Input: part model. Units: mm. Frame: model coordinates. A direction names the side the tool comes from. Round coordinates to 2 decimals unless told otherwise and drop trailing zeros. Write each loop counter-clockwise with the first axis right and the second up, starting at its lowest first coordinate (ties: lowest second). Pieces come first, ordered by that corner, then holes. Notation, with made-up numbers: (31, 72.5) -> (77, 72.5) arc R26 ccw to (77, 108.5) -> close; hole circle Ø4 at (15.25, 32). An arc over 180 degrees is marked (long way). Write item = value, one per line. Start each with the question number.
Autodesk Inventor part; units mm, degrees
ref_plane "YZ Plane" through (0, 0, 0) normal (1, 0, 0) x (0, 1, 0)
ref_plane "XZ Plane" through (0, 0, 0) normal (0, 1, 0) x (-1, 0, 0)
ref_plane "XY Plane" through (0, 0, 0) normal (0, 0, 1) x (1, 0, 0)
sketch "Skizze1" plane through (0, 0, 0) normal (0, 0, 1) x (1, 0, 0)
  circle A0 centre (0, 0) radius 12.5
  dimension "d0" = 25
extrude "Extrusion1" add sketch "Skizze1" along normal blind 4
sketch "Skizze2" plane through (0, 0, 4) normal (0, 0, 1) x (1, 0, 0)
  circle A0 centre (0, 0) radius 12.5
  circle A1 centre (0, 0) radius 5.5
  dimension "d3" = 11
extrude "Extrusion2" add sketch "Skizze2" along normal blind 9 contours A1
sketch "Skizze3" plane through (0, 0, 13) normal (0, 0, 1) x (1, 0, 0)
  circle A0 centre (0, 0) radius 5.5
  circle A1 centre (0, 0) radius 4
  dimension "d6" = 8
extrude "Extrusion3" add sketch "Skizze3" along normal blind 9 contours A1
sketch "Skizze4" plane through (0, 0, 0) normal (0, 0, -1) x (-1, 0, 0)
  circle A0 centre (0, 0) radius 12.5
  line L0 (17.5, 0) -> (-17.5, 0)
  line L1 (0, -17.5) -> (0, 17.5)
  circle A1 centre (0, 0) radius 9
  line L2 (7.7942, -4.5) -> (0, 0)
  line L3 (0, 0) -> (-7.7942, -4.5)
  point P0 (0, 9)
  dimension "d9" = 18
  dimension "d10" = 120
  dimension "d11" = 120
hole "Bohrung1" at (0, 9, 0) at (-7.7942, -4.5, 0) at (7.7942, -4.5, 0) direction (0, 0, 1) diameter 2.459 end through all
chamfer "Fase1" distance 0.5 angle 45 1 edges at (-4, 0, 22)
sketch "Skizze5" plane through (0, 0, 0) normal (1, 0, 0) x (0, 1, 0)
  line L0 (-4, 13) -> (4, 13)
  line L1 (4, 21.5) -> (-4, 21.5)
  line L2 (4, 13) -> (4, 21.5)
  line L3 (0, -4.3) -> (0, 25.8)
  line L4 (4, 20.9) -> (3.8, 20.9)
  line L5 (3.8, 20.9) -> (3.8, 20)
  line L6 (3.8, 20) -> (4, 20)
  line L7 (4, 20) -> (4, 20.9)
  point P0 (0, 0)
  dimension "d31" = 7
  dimension "d32" = 0.9
  dimension "d33" = 7.6
revolve "Umdrehung1" cut sketch "Skizze5" angle 360 about axis through (0, 0, -10) along (0, 0, 1) contours L6 L5 L4 L2
chamfer "Fase3" distance 1 angle 45 1 edges at (-12.5, 0, 4)
properties part number "1_0204_005"
1. Section D-D (y = -4.5). State how many separate pieces and enclosed holes the cut face has, then the cut area to 3 significant figures.
2. Section C-C (z = 16.75). Output: boundary loops of the cut face in (x, y).
3. Line query: line 1 along Y through (x, z) = (0, 1.6); line 2 along X through (y, z) = (-4.5, 1.6); line 3 along Z through (x, y) = (0.5, 7). Output: solid intervals per line, ascending.
4. Section B-B (y = 0). Output: boundary loops of the cut face in (x, z).
5. Pin query (flat end, axial travel): P1, Ø3, axis at x = 7.79, y = -4.5, coming from the +Z side; P2, Ø1, axis at x = -1.5, z = 14.5, coming from the -Y side; P3, Ø3, axis at x = -2.5, z = 11, coming from the +Y side. Return the tip coordinate at first contact, or that it passes through.
6. Mould query, pull axis Y, two halves, no side actions, for faces 1 (the flat face through (0, 0, 0)), 2 (the cylindrical face through (-8.625, -5.406, 2.028)), 3 (the cylindrical face through (0.167, -3.796, 20.444)). Classes: pulls with the +Y half, pulls with the -Y half, needs draft (parallel to the pull), parting line crosses it, or undercut.
7. Section A-A (x = 0). Output: boundary loops of the cut face in (y, z), then the cut area to 3 significant figures.
8. Reachability of faces 4 (the cylindrical face through (6.963, -5.406, 2.028)), 5 (the cylindrical face through (-0.867, 3.905, 16.451)) from +Z, -Z, +X, -X, +Y, -Y: full face, straight path, thin tool, end or side. Return the list, or none.
Check sheet entries:
q1.separate_pieces = 3
q1.enclosed_holes = 0
q1.area = 129 mm2
q2.outline = circle Ø8 at (0, 0)
q3.line_1 = -12.5 to 7.77, 10.23 to 12.5
q3.line_2 = -11.66 to -9.02, -6.56 to 6.56, 9.02 to 11.66
q3.line_3 = 0 to 4
q4.outline = (-12.5, 0) -> (12.5, 0) -> (12.5, 3) -> (11.5, 4) -> (5.5, 4) -> (5.5, 13) -> (4, 13) -> (4, 20) -> (3.8, 20) -> (3.8, 20.9) -> (4, 20.9) -> (4, 21.5) -> (3.5, 22) -> (-3.5, 22) -> (-4, 21.5) -> (-4, 20.9) -> (-3.8, 20.9) -> (-3.8, 20) -> (-4, 20) -> (-4, 13) -> (-5.5, 13) -> (-5.5, 4) -> (-11.5, 4) -> (-12.5, 3) -> close
q5.P1 = 4
q5.P2 = -3.87
q5.P3 = 5.41
q6.face_1 = needs draft
q6.face_2 = undercut
q6.face_3 = parting line crosses it
q7.outline = (-12.5, 0) -> (7.77, 0) -> (7.77, 4) -> (5.5, 4) -> (5.5, 13) -> (4, 13) -> (4, 20) -> (3.8, 20) -> (3.8, 20.9) -> (4, 20.9) -> (4, 21.5) -> (3.5, 22) -> (-3.5, 22) -> (-4, 21.5) -> (-4, 20.9) -> (-3.8, 20.9) -> (-3.8, 20) -> (-4, 20) -> (-4, 13) -> (-5.5, 13) -> (-5.5, 4) -> (-11.5, 4) -> (-12.5, 3) -> close; (10.23, 0) -> (12.5, 0) -> (12.5, 3) -> (11.5, 4) -> (10.23, 4) -> close
q7.area = 260 mm2
q8.face_4 = +Z, -Z
q8.face_5 = +Z
